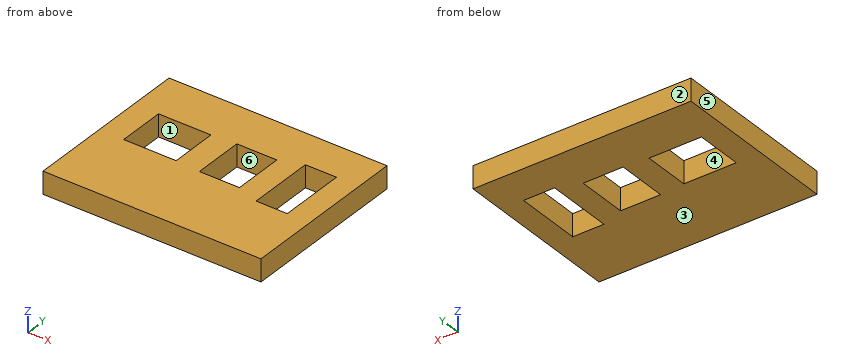
from build123d import *

# Parameters (mm, degrees)
F0_W     = 245
F0_H     = 160
F0_W_2   = 59
F0_H_2   = 53
F0_W_3   = 45
F0_H_3   = 57
F0_W_4   = 35
F0_H_4   = 75
F0_H_5   = 32
F1_DEPTH = 25


with BuildPart() as f1:
    # F0 (on Top) → F1 (new body)
    with BuildSketch(Plane.XY):
        Rectangle(F0_W, F0_H)
        with Locations((-65.4, 0)):
            Rectangle(F0_W_2, F0_H_2, mode=Mode.SUBTRACT)
        with Locations((14.2, 0)):
            Rectangle(F0_W_3, F0_H_3, mode=Mode.SUBTRACT)
        with Locations((79.6, 0)):
            Rectangle(F0_W_4, F0_H_4, mode=Mode.SUBTRACT)
        with Locations((0, -96)):
            Rectangle(F0_W, F0_H_5)
    extrude(amount=F1_DEPTH)


solid = f1.part
Can you work these out from the model? Positions are in its coordinate system, mm. Face numbers are marked on the shaded views. A direction names the side the tool comes from. Coordinates: 2 decimals unless noted, no trailing zeros. Order: outer loops, then holes, each group sorted by start corner. A loop starts at its lowest first (then second) coordinate and runs counter-clockwise, first axis right, second up. Notation, with made-up numbers: (67.5, 64.25) - (73.5, 64.25) arc R24 cw to (73.5, 92.25) - close; hole circle Ø11 at (76, 89.25). An arc over 180 degrees is marked (long way). Answer as a JSON object with one key per item and string values. Group by question number.
Q1. We'd pull the mould along X, two halves only. Please class the marked faces 3, 4, 5 and 6: +X half, -X half, draft (parallel to the pull), parting line (faces both ways), or undercut.
Q2. Imagine slicing it at B-B (x = -48.5). Please give me the cut outline in (y, z).
Q3. On a 3-axis mill with a long thin cutter (end or side, diameter ignored), from which of +Z, -Z, +X, -X, +Y, -Y can I reach the whole of each face in a straight line? I mean the marked faces 1 and 2. Say none if no direction works.
Q4. Imagine slicing it at A-A (z = 16.25). Please give me the cut outline in (x, y).
Q5. Imagine slicing it at C-C (x = 8). Please give me the cut outline in (y, z), and give its area (4 significant figures).
Q6. I need wall thicknesses on line 1 (X direction, y = -4.5, z = 2.75); line 2 (Y direction, x = 70, z = 11.25); line 3 (Y direction, x = -66.5, z = 7.5). Which ranges of each line are inside material? Lowest first, please. Write a range as from..to.
Determined:
{
 "1": {"face 3": "draft", "face 4": "undercut", "face 5": "-X half", "face 6": "undercut"},
 "2": {"outline": "(-112, 0) - (-26.5, 0) - (-26.5, 25) - (-112, 25) - close; (26.5, 0) - (80, 0) - (80, 25) - (26.5, 25) - close"},
 "3": {"face 1": "+Z, -Z", "face 2": "+Z, -Z, +X, -X, +Y"},
 "4": {"outline": "(-122.5, -112) - (122.5, -112) - (122.5, 80) - (-122.5, 80) - close; hole (-94.9, -26.5) - (-35.9, -26.5) - (-35.9, 26.5) - (-94.9, 26.5) - close; hole (-8.3, -28.5) - (36.7, -28.5) - (36.7, 28.5) - (-8.3, 28.5) - close; hole (62.1, -37.5) - (97.1, -37.5) - (97.1, 37.5) - (62.1, 37.5) - close"},
 "5": {"outline": "(-112, 0) - (-28.5, 0) - (-28.5, 25) - (-112, 25) - close; (28.5, 0) - (80, 0) - (80, 25) - (28.5, 25) - close", "area": "3,375 mm2"},
 "6": {"line 1": "x = -122.5..-94.9, -35.9..-8.3, 36.7..62.1, 97.1..122.5", "line 2": "y = -112..-37.5, 37.5..80", "line 3": "y = -112..-26.5, 26.5..80"}
}
